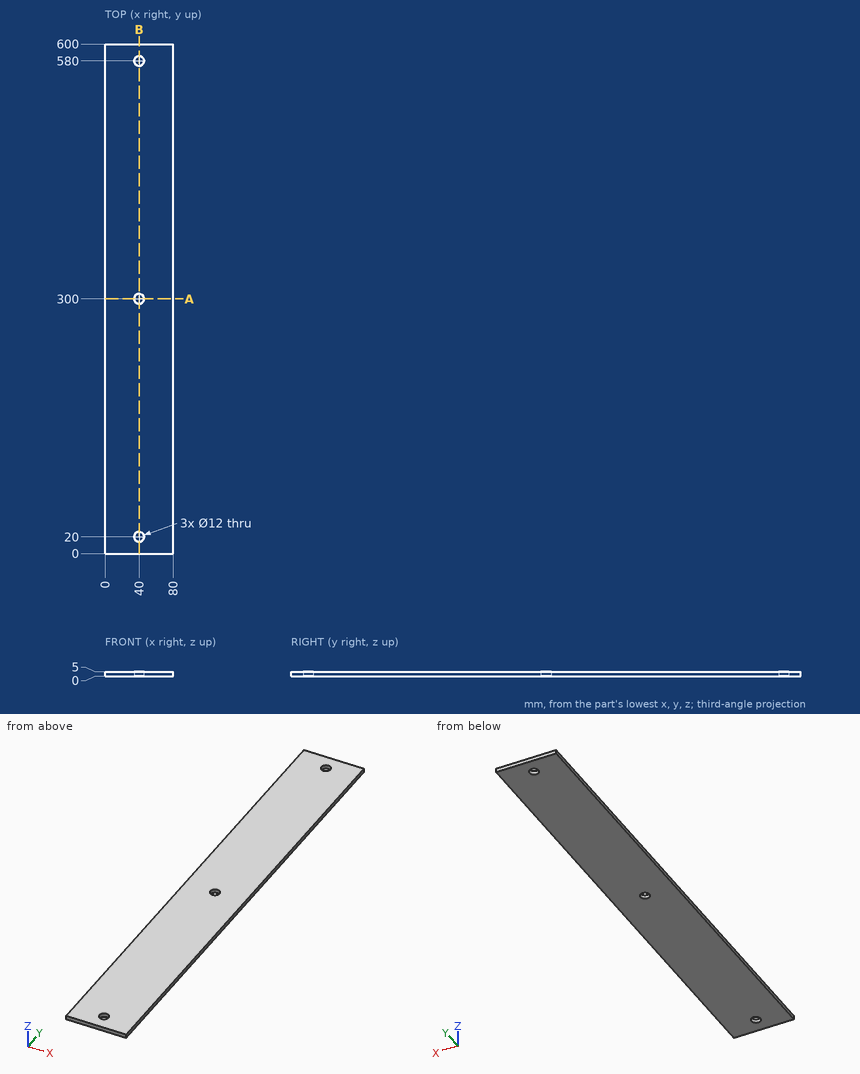
Geometry check sheet. Reference: drawing and pictorial views, mm from the part's lowest x, y, z. Coordinates: 2 decimals unless noted, no trailing zeros. Order: outer loops, then holes, each group sorted by start corner. A loop starts at its lowest first (then second) coordinate and runs counter-clockwise, first axis right, second up.
Item 1: Section check B-B, the plane x = 40. Enter the section's corners in (y, z).
Filled in:
outline: (0, 0) - (14, 0) - (14, 5) - (0, 5) - close; (26, 0) - (294, 0) - (294, 5) - (26, 5) - close; (306, 0) - (574, 0) - (574, 5) - (306, 5) - close; (586, 0) - (600, 0) - (600, 5) - (586, 5) - close
Item 2: Material ranges on L1, parallel to Y at x = 40, z = 3.4; L2, parallel to X at y = 20, z = 1.2; L3, parallel to Y at x = 41.5, z = 3.7, recorded low to high.
Filled in:
L1: y = 0 to 14, 26 to 294, 306 to 574, 586 to 600
L2: x = 0 to 34, 46 to 80
L3: y = 0 to 14.19, 25.81 to 294.19, 305.81 to 574.19, 585.81 to 600
Item 3: Section check A-A, the plane y = 300. Enter the section's corners in (x, z), then the cut area to 3 significant figures.
Filled in:
outline: (0, 0) - (34, 0) - (34, 5) - (0, 5) - close; (46, 0) - (80, 0) - (80, 5) - (46, 5) - close
area: 340 mm2
Item 4: Depth check by flat-ended pin: pin 1 (19 mm diameter, centred on x = 40, y = 580, fed in from +Z); pin 2 (11 mm diameter, centred on x = 40, y = 300, fed in from -Z). Enter the tip coordinate at first touch or a pass-through.
Filled in:
pin 1: stops at z = 5
pin 2: passes through
